Here's how the part is built. I have some questions about the finished solid (model axes, mm). Face numbers are marked on the shaded views. A direction names the side the tool comes from. Coordinates: 2 decimals unless noted, no trailing zeros. Order: outer loops, then holes, each group sorted by start corner. A loop starts at its lowest first (then second) coordinate and runs counter-clockwise, first axis right, second up. Notation, with made-up numbers: (78.25, 71.5) - (125.25, 71.5) arc R15 ccw to (125.25, 75.5) - close; hole circle Ø8 at (-1, -11). An arc over 180 degrees is marked (long way). Answer as CSV lines item,"result". Start each with the question number.
Q1. I need wall thicknesses on line 1 (Y direction, x = 3.25, z = -9); line 2 (Z direction, x = 7.5, y = -6); line 3 (Z direction, x = 8.5, y = 26). Which ranges of each line are inside material? Lowest first, please.
Q2. Suppose I cut it at B-B (z = -4). Please give me the cut outline in (x, y), then the cut area to 3 significant figures.
Q3. Suppose I cut it at D-D (z = 18.5). Please give me the cut outline in (x, y).
Q4. Thinking about a two-plate mould opening in X: for the marked faces 1, 2 and 3, which applies, released by +X, released by -X, zero draft, split by the parting line, or undercut?
Q5. Suppose I cut it at C-C (y = 13). Please give me the cut outline in (x, z), then the cut area to 3 significant figures.
Q6. Suppose I cut it at A-A (x = 5.75). Please give me the cut outline in (y, z).
Q7. For the marked faces 4, 5 and 6, which set-ups out of +Z, -Z, +X, -X, +Y, -Y let a thin tool reach every point of the face, with its end or its side?
Q8. For pin 1 Ø1.5 at (x, z) = (5, 12) entering from -Y; pin 2 Ø3 at (x, y) = (8.5, 36) entering from +Z; pin 3 Ø2.5 at (y, z) = (29.5, -15) entering from +X, each with a flat end and sliding along its axis, tell me the tip position at first contact or that it passes through.
from build123d import *

# Parameters (mm, degrees)
SKETCH1_R           = 1.5
BOSS_EXTRUDE1_DEPTH = 10
FILLET1_R           = 1
SKETCH2_W           = 5
SKETCH2_H           = 7
CUT_EXTRUDE1_DEPTH  = 7
FILLET3_R           = 2
CUT_EXTRUDE2_DEPTH  = 20
SKETCH4_W           = 5
SKETCH4_H           = 17.5
BOSS_EXTRUDE3_DEPTH = 5


with BuildPart() as part:
    # Sketch1 → Boss-Extrude1 (new body)
    with BuildSketch(Plane(origin=(0, 0, 0), x_dir=(0, 0, -1), z_dir=(1, 0, 0))):
        Polygon((-37.823529412, -17.294117647), (-22.823529412, -17.294117647), (-2.823529412, -7.294117647), (7.176470588, 32.705882353), (7.176470588, 39.705882353), (0.176470588, 39.705882353), (0.176470588, 32.705882353), (-9.823529412, -2.294117647), align=None)
        with Locations((3.676470588, 36.205882353)):
            Circle(SKETCH1_R, mode=Mode.SUBTRACT)
        with Locations((-6.323529412, -2.294117647)):
            Circle(SKETCH1_R, mode=Mode.SUBTRACT)
    extrude(amount=BOSS_EXTRUDE1_DEPTH)

    # Fillet1
    fillet1_edges = [part.edges().sort_by_distance(p)[0] for p in [
        (5, -17.294117647, 37.823529412),
    ]]
    fillet(fillet1_edges, radius=FILLET1_R)

    # Sketch2 → Cut-Extrude1 (cut)
    with BuildSketch(Plane(origin=(0, 39.705882353, 0), x_dir=(1, 0, 0), z_dir=(0, 1, 0))):
        with Locations((5, 3.676470588)):
            Rectangle(SKETCH2_W, SKETCH2_H)
    extrude(amount=-CUT_EXTRUDE1_DEPTH, mode=Mode.SUBTRACT)

    # Fillet3
    fillet3_edges = [part.edges().sort_by_distance(p)[0] for p in [
        (8.75, 39.705882353, -0.176470588),
        (8.75, 39.705882353, -7.176470588),
        (1.25, 39.705882353, -0.176470588),
        (1.25, 39.705882353, -7.176470588),
        (5, 32.705882353, -0.176470588),
    ]]
    fillet(fillet3_edges, radius=FILLET3_R)

    # Sketch3 → Cut-Extrude2 (cut)
    with BuildSketch(Plane(origin=(10, 0, 0), x_dir=(0, 0, -1), z_dir=(1, 0, 0))):
        Polygon((-33.839212055, -17.294117647), (-2.823529412, -7.294117647), (-22.823529412, -17.294117647), align=None)
    extrude(amount=-CUT_EXTRUDE2_DEPTH, mode=Mode.SUBTRACT)

    # Sketch4 → Boss-Extrude3 (add)
    with BuildSketch(Plane(origin=(0, 32.705882353, 0), x_dir=(1, 0, 0), z_dir=(0, 1, 0))):
        with Locations((5, 10.435073414)):
            Rectangle(SKETCH4_W, SKETCH4_H)
    extrude(amount=-BOSS_EXTRUDE3_DEPTH)


solid = part.part
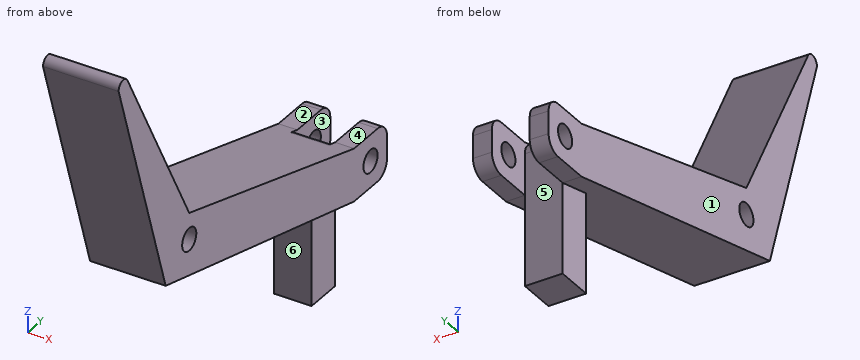
Here are the results:
1,line 1,"y = 27.71 to 32.71"
1,line 2,"z = 2.5 to 16.74"
1,line 3,"z = -5.5 to 1.74"
2,outline,"(0, 20) - (10, 20) - (10, 34.74) - (7.5, 34.74) - (7.5, 32.71) - (2.5, 32.71) - (2.5, 34.74) - (0, 34.74) - close; (0, 37.67) - (2.5, 37.67) - (2.5, 39.71) - (0, 39.71) - close; (7.5, 37.67) - (10, 37.67) - (10, 39.71) - (7.5, 39.71) - close"
2,area,"147 mm²"
3,outline,"(0, -12.35) - (10, -12.35) - (10, -6.94) - (0, -6.94) - close"
4,face 1,"released by -X"
4,face 2,"zero draft"
4,face 3,"undercut"
5,outline,"(0, -2.25) - (10, -2.25) - (10, 5.45) - (0, 5.45) - close"
5,area,"77.0 mm²"
6,outline,"(-17.29, 33.84) - (-7.29, 2.82) - (27.71, -5.93) - (27.71, -19.19) - (32.71, -19.19) - (32.71, -1.69) arc R2 ccw to (31.26, 0.24) - (-2.29, 9.82) - (-15.41, 34.31) arc R1 ccw to start; hole circle Ø3 at (-2.29, 6.32)"
7,face 4,"+Z, +X, -X, +Y"
7,face 5,"+Z, -Z, +Y"
7,face 6,"-Z, +X, -X, -Y"
8,pin 1,"stops at y = -10.49"
8,pin 2,"stops at z = -0.18"
8,pin 3,"stops at x = 7.5"
